Geometry: final body of the model. Coordinates: model frame, mm. Round coordinates to 2 decimals unless told otherwise and drop trailing zeros. Order: outer loops, then holes, each group sorted by start corner. A loop starts at its lowest first (then second) coordinate and runs counter-clockwise, first axis right, second up. Notation, with made-up numbers: M 4,76.25 L 46,76.25 A20 ccw 46,93.25 Z; hole C 64.25,-15.75 d5. An arc over 180 degrees is marked long. Put each result on its own line as item: value. Start each with the question number.
1) First-contact query: P1, Ø4, axis at x = -4, y = -7, coming from the -Z side. Flat tip, straight axial feed; report the tip coordinate or a pass-through.
2) Section A-A, the plane y = 0. Return loops of the section in (x, z).
3) Draft query along Y for faces 1 (the cylindrical face through (-0.867, -3.905, 6.084)), 2 (the flat face through (10, -4, 6)), 3 (the flat face through (0, -9, 6)). Return one class per face: pulls with the +Y half, pulls with the -Y half, needs draft (parallel to the pull), parting line crosses it, or undercut.
4) Material intervals for probe 1 along Y at (x, z) = (9, 3); probe 2 along Y at (x, z) = (0, 5); probe 3 along X at (y, z) = (-3.5, 9.5), sorted ascending. Write a range as [from, to].
5) Section C-C, the plane z = 2.75. Return loops of the section in (x, y).
6) Section B-B, the plane x = 9. Return loops of the section in (y, z), then the cut area to 3 significant figures.
from build123d import *

# Parameters (mm, degrees)
SKETCH1_W           = 20
SKETCH1_H           = 18
BOSS_EXTRUDE1_DEPTH = 12
SKETCH2_R           = 1.5
SKETCH2_R_2         = 4
CUT_EXTRUDE1_DEPTH  = 13
CHAMFER1_SIZE       = 2


with BuildPart() as part:
    # Sketch1 → Boss-Extrude1 (new body)
    with BuildSketch(Plane.XY):
        Rectangle(SKETCH1_W, SKETCH1_H)
    extrude(amount=BOSS_EXTRUDE1_DEPTH)

    # Sketch2 → Cut-Extrude1 (cut, through all)
    with BuildSketch(Plane.XY.offset(12)):
        with Locations((9, 0)):
            Circle(SKETCH2_R)
        Circle(SKETCH2_R_2)
    extrude(amount=-CUT_EXTRUDE1_DEPTH, mode=Mode.SUBTRACT)

    # Chamfer1
    chamfer1_edges = [part.edges().sort_by_distance(p)[0] for p in [
        (10, 9, 6),
        (10, -9, 6),
        (-10, -9, 6),
        (-10, 9, 6),
    ]]
    chamfer(chamfer1_edges, length=CHAMFER1_SIZE)


solid = part.part
Result sheet:
1. P1: stops at z = 0
2. outline: M -10,0 L -4,0 L -4,12 L -10,12 Z; M 4,0 L 7.5,0 L 7.5,12 L 4,12 Z
3. face 1: undercut
3. face 2: needs draft
3. face 3: pulls with the -Y half
4. probe 1: y = [-8, -1.5], [1.5, 8]
4. probe 2: y = [-9, -4], [4, 9]
4. probe 3: x = [-10, -1.94], [1.94, 10]
5. outline: M -10,-7 L -8,-9 L 8,-9 L 10,-7 L 10,-1.12 A1.5 cw long 10,1.12 L 10,7 L 8,9 L -8,9 L -10,7 Z; hole C 0,0 d8
6. outline: M -8,0 L -1.5,0 L -1.5,12 L -8,12 Z; M 1.5,0 L 8,0 L 8,12 L 1.5,12 Z
6. area: 156 mm2
